```python
from build123d import *

# Parameters (mm, degrees)
CROQUIS1_R              = 50
CROQUIS1_R_2            = 4
SALIENTE_EXTRUIR3_DEPTH = 3


with BuildPart() as part:
    # Croquis1 → Saliente-Extruir3 (new body)
    with BuildSketch(Plane.XY):
        Circle(CROQUIS1_R)
        Circle(CROQUIS1_R_2, mode=Mode.SUBTRACT)
        with BuildLine():
            ThreePointArc((0.780784951, 45.593315024), (0.000190465, 46.806858641), (0.821878896, 47.992963183))
            ThreePointArc((0.821878896, 47.992963183), (15.980042003, 45.261885263), (29.492838566, 37.870469674))
            ThreePointArc((29.492838566, 37.870469674), (29.647643774, 36.228936164), (28.018196638, 35.97694619))
            ThreePointArc((28.018196638, 35.97694619), (15.181039903, 42.998791), (0.780784951, 45.593315024))
        make_face(mode=Mode.SUBTRACT)
        with BuildLine():
            ThreePointArc((35.97694619, -28.018196638), (42.998791, -15.181039903), (45.593315024, -0.780784951))
            ThreePointArc((45.593315024, -0.780784951), (46.806858641, -0.000190465), (47.992963183, -0.821878896))
            ThreePointArc((47.992963183, -0.821878896), (45.261885263, -15.980042003), (37.870469674, -29.492838566))
            ThreePointArc((37.870469674, -29.492838566), (36.228936164, -29.647643774), (35.97694619, -28.018196638))
        make_face(mode=Mode.SUBTRACT)
        with BuildLine():
            ThreePointArc((-28.018196638, -35.97694619), (-15.181039903, -42.998791), (-0.780784951, -45.593315024))
            ThreePointArc((-0.780784951, -45.593315024), (-0.000190465, -46.806858641), (-0.821878896, -47.992963183))
            ThreePointArc((-0.821878896, -47.992963183), (-15.980042003, -45.261885263), (-29.492838566, -37.870469674))
            ThreePointArc((-29.492838566, -37.870469674), (-29.647643774, -36.228936164), (-28.018196638, -35.97694619))
        make_face(mode=Mode.SUBTRACT)
        with BuildLine():
            ThreePointArc((-35.97694619, 28.018196638), (-42.998791, 15.181039903), (-45.593315024, 0.780784951))
            ThreePointArc((-45.593315024, 0.780784951), (-46.806858641, 0.000190465), (-47.992963183, 0.821878896))
            ThreePointArc((-47.992963183, 0.821878896), (-45.261885263, 15.980042003), (-37.870469674, 29.492838566))
            ThreePointArc((-37.870469674, 29.492838566), (-36.228936164, 29.647643774), (-35.97694619, 28.018196638))
        make_face(mode=Mode.SUBTRACT)
        with BuildLine():
            ThreePointArc((42.238881445, -14.930401679), (40.398847807, 19.364222056), (14.817024573, 42.27878644))
            ThreePointArc((14.817024573, 42.27878644), (13.287672492, 41.543203533), (14.023255399, 40.013851452))
            ThreePointArc((14.023255399, 40.013851452), (38.234623818, 18.326853017), (39.976084224, -14.130558732))
            ThreePointArc((39.976084224, -14.130558732), (40.707561361, -15.661878816), (42.238881445, -14.930401679))
        make_face(mode=Mode.SUBTRACT)
        with BuildLine():
            ThreePointArc((-39.976084224, 14.130558732), (-38.234623818, -18.326853017), (-14.023255399, -40.013851452))
            ThreePointArc((-14.023255399, -40.013851452), (-13.287672492, -41.543203533), (-14.817024573, -42.27878644))
            ThreePointArc((-14.817024573, -42.27878644), (-40.398847807, -19.364222056), (-42.238881445, 14.930401679))
            ThreePointArc((-42.238881445, 14.930401679), (-40.707561361, 15.661878816), (-39.976084224, 14.130558732))
        make_face(mode=Mode.SUBTRACT)
        with BuildLine():
            ThreePointArc((-36.967560027, -17.263820715), (17.510315589, -36.851442957), (36.733682313, 17.756029503))
            ThreePointArc((36.733682313, 17.756029503), (35.13104373, 18.314195762), (34.572877471, 16.711557179))
            ThreePointArc((34.572877471, 16.711557179), (16.480297025, -34.683711018), (-34.792997672, -16.248301849))
            ThreePointArc((-34.792997672, -16.248301849), (-36.388038282, -15.668780105), (-36.967560027, -17.263820715))
        make_face(mode=Mode.SUBTRACT)
        with BuildLine():
            ThreePointArc((-14.023255399, 34.023349453), (-33.48596426, -15.262050897), (16.480297025, -32.903492368))
            ThreePointArc((16.480297025, -32.903492368), (17.015836003, -31.293151409), (15.405495045, -30.75761243))
            ThreePointArc((15.405495045, -30.75761243), (-31.302097025, -14.266699752), (-13.108695264, 31.804435358))
            ThreePointArc((-13.108695264, 31.804435358), (-12.456518284, 33.371172473), (-14.023255399, 34.023349453))
        make_face(mode=Mode.SUBTRACT)
    extrude(amount=SALIENTE_EXTRUIR3_DEPTH)


solid = part.part
```
For this review, take the finished solid that the model builds, in its own axes (mm). Round coordinates to 2 decimals unless told otherwise and drop trailing zeros. Order: outer loops, then holes, each group sorted by start corner. A loop starts at its lowest first (then second) coordinate and runs counter-clockwise, first axis right, second up. Notation, with made-up numbers: (-19, -8) -> (39, -8) arc R10 cw to (39, 11) -> close; hole circle Ø5 at (-25, 83). An arc over 180 degrees is marked (long way). Use a Markdown table: item, result.
Item 1: For pin 1 (1 mm diameter, centred on x = 11, z = 2.5, fed in from -Y), flat-tipped, find the tip position at first contact; note if it passes through.
Resolved:
| item | result |
|---|---|
| pin 1 | stops at y = -48.89 |
Item 2: Take a section at A-A (y = -22.5). State the section outline as (x, z) points.
Resolved:
| item | result |
|---|---|
| outline | (-44.65, 0) -> (-38.74, 0) -> (-38.74, 3) -> (-44.65, 3) -> close; (-35.94, 0) -> (-34.04, 0) -> (-34.04, 3) -> (-35.94, 3) -> close; (-31.12, 0) -> (-29.12, 0) -> (-29.12, 3) -> (-31.12, 3) -> close; (-26.02, 0) -> (31.12, 0) -> (31.12, 3) -> (-26.02, 3) -> close; (34.04, 0) -> (39.66, 0) -> (39.66, 3) -> (34.04, 3) -> close; (42.4, 0) -> (44.65, 0) -> (44.65, 3) -> (42.4, 3) -> close |
Item 3: For line 1 along Y through (x, z) = (-16, 2.95); line 2 along Y through (x, z) = (-11.5, 2.75); line 3 along X through (y, z) = (41.5, 2.65), list the stretches that pass through material, from the lowest coordinate up. Write a range as [from, to].
Resolved:
| item | result |
|---|---|
| line 1 | y = [-47.37, -45.25], [-42.7, -41.85], [-39.27, -37.53], [-34.91, -33.14], [-30.45, 30.45], [33.14, 47.37] |
| line 2 | y = [-48.66, -46.6], [-44.13, -39.15], [-36.64, -34.96], [-32.42, 48.66] |
| line 3 | x = [-27.89, 13.27], [16.88, 18.9], [24.12, 27.89] |
Item 4: Take a section at B-B (x = -33). State the section outline as (y, z) points, plus the area to 3 significant figures.
Resolved:
| item | result |
|---|---|
| outline | (-37.56, 0) -> (-30.3, 0) -> (-30.3, 3) -> (-37.56, 3) -> close; (-26.62, 0) -> (-23.99, 0) -> (-23.99, 3) -> (-26.62, 3) -> close; (-19.64, 0) -> (-16.29, 0) -> (-16.29, 3) -> (-19.64, 3) -> close; (-9.71, 0) -> (9.71, 0) -> (9.71, 3) -> (-9.71, 3) -> close; (16.29, 0) -> (37.56, 0) -> (37.56, 3) -> (16.29, 3) -> close |
| area | 162 mm² |
Item 5: Take a section at C-C (z = 2.3). State how many separate pieces and enclosed holes the cut face has, plus the area to 3 significant figures.
Resolved:
| item | result |
|---|---|
| separate pieces | 1 |
| enclosed holes | 9 |
| area | 6,580 mm² |
Item 6: Draft analysis for pull direction Y (two halves, no side actions). For faces 1 (the cylindrical face through (17.242, -34.311, 1.479)), 2 (the cylindrical face through (47.69, 15.02, 1.48)), 3 (the flat face through (10, 1, 0)), state which applies: +Y half, -Y half, draft (parallel to the pull), parting line (faces both ways), or undercut.
Resolved:
| item | result |
|---|---|
| face 1 | undercut |
| face 2 | parting line |
| face 3 | draft |
